Geometry check sheet. Reference: the model listing, model coordinates, mm. A direction names the side the tool comes from. Give positions to 0.01 mm unless a question says otherwise; leave off trailing zeros. Write each loop counter-clockwise with the first axis right and the second up, starting at its lowest first coordinate (ties: lowest second). Pieces come first, ordered by that corner, then holes. Notation, with made-up numbers: M 42.25,-12 L 81.25,-12 A30 cw 81.25,15 Z; hole C 3.5,69.25 d4. An arc over 180 degrees is marked long. One line per item, written item: value. Start each with the question number.
1. Cross-section at A-A on z = 7. Record the cut outline in (x, y).
2. Cross-section at B-B on z = -1.5. Record the cut outline in (x, y).
3. Gauge pin test, flat ends, axial feed: pin 1 (3 mm diameter, centred on y = 48, z = 32, fed in from +X); pin 2 (0.5 mm diameter, centred on x = -1.5, y = 49, fed in from -Z); pin 3 (1.5 mm diameter, centred on y = 50, z = 25, fed in from -X). Record the tip position at first contact, or that the pin passes through.
4. Scan lines: line 1 (Z direction, x = -1.45, y = 48); line 2 (X direction, y = 46.5, z = -1.5); line 3 (Z direction, x = -3.3, y = 48.25). Record each from-to range of solid material in increasing order.
5. Tool access check on faces 1 (the face through (-3.62, 48, -3)), 2 (the face through (-1.968, 48, -3)), 3 (the face through (-3, 50.8, 16)). Record the directions out of +Z, -Z, +X, -X, +Y, -Y that give a thin tool (end or side, any length) a straight path to the whole face; none if there is none.
Autodesk Inventor part; units mm, degrees
ref_plane "Work Plane1" through (0, 50.8, 0) normal (0, 1, 0) x (-1, 0, 0)
ref_plane "YZ Plane" through (0, 0, 0) normal (1, 0, 0) x (0, 1, 0)
ref_plane "XY Plane" through (0, 0, 0) normal (0, 0, 1) x (1, 0, 0)
sketch "Sketch6" plane through (0, 0, 0) normal (0, 1, 0) x (-1, 0, 0)
  line L0 (0, 0) -> (5.588, 0)
  line L1 (5.588, 0) -> (5.588, -6.35)
  line L2 (5.588, -6.35) -> (0, -6.35)
  line L3 (0, -6.35) -> (0, 0)
  arc A0 (0, -6.35) -> (5.588, -6.35) centre (2.794, -6.35) ccw
  dimension "d25" = 5.588
  dimension "d26" = 6.35
ref_plane "Work Plane1" through (0, 50.8, 0) normal (0, 1, 0) x (-1, 0, 0)
sketch "Sketch8" plane through (0, 50.8, 0) normal (0, 1, 0) x (-1, 0, 0)
  line L0 (4.3815, 0) -> (1.2065, 0)
  line L1 (1.2065, 0) -> (1.2065, -3.81)
  line L2 (1.2065, -3.81) -> (4.3815, -3.81)
  line L3 (4.3815, -3.81) -> (4.3815, 0)
  arc A0 (1.2065, -3.81) -> (4.3815, -3.81) centre (2.794, -3.81) ccw
  point P0 (0, 0)
  dimension "d27" = 3.175
  dimension "d28" = 3.81
  dimension "d49" = 1.2065
loft "Loft1" add profiles "Sketch6", "Sketch8"
sketch "Sketch9" plane through (-5.588, 0, 0) normal (0, 0, 1) x (1, 0, 0)
  line L0 (0, 0) -> (5.588, 0)
  line L1 (5.588, 0) -> (4.3815, 50.8)
  line L2 (1.2065, 50.8) -> (4.3815, 50.8)
  line L3 (0, 0) -> (1.2065, 50.8)
  line L4 (4.3815, 50.8) -> (5.588, 0)
  line L5 (4.5323, 44.45) -> (1.0557, 44.45)
  line L6 (0, 0) -> (1.2065, 50.8)
  dimension "d34" = 6.35
extrude "Extrusion5" add sketch "Sketch9" along normal blind 38.608 contours L3 L2 L1 L5
sketch "Sketch12" plane through (-2.794, 0, -6.35) normal (0, -1, 0) x (1, 0, 0)
  circle A0 centre (0, 1.9685) radius 1.27
  arc A1 (-2.794, 0) -> (2.794, 0) centre (0, 0) ccw
  line L0 (0, -2.794) -> (0, 1.9685)
  point P0 (2.794, 6.35)
  dimension "d44" = 2.54
  dimension "d46" = 4.7625
extrude "Extrusion8" cut sketch "Sketch12" against normal blind 10.16
sketch "Sketch13" plane through (-5.588, 0, 0) normal (0, 0, 1) x (1, 0, 0)
  line L0 (4.3815, 50.8) -> (1.2065, 50.8)
  line L1 (1.2065, 50.8) -> (4.3815, 50.8)
  line L2 (1.0557, 44.45) -> (4.5323, 44.45)
  line L3 (3.6195, 50.8) -> (1.9685, 50.8)
  line L4 (1.9685, 50.8) -> (1.9685, 44.45)
  line L5 (1.9685, 44.45) -> (3.6195, 44.45)
  line L6 (3.6195, 44.45) -> (3.6195, 50.8)
  line L7 (3.6195, 50.8) -> (4.3815, 50.8) construction
  line L8 (0, 0) -> (1.2065, 50.8) construction
  line L9 (1.9685, 50.8) -> (1.2065, 50.8) construction
  line L10 (10.7022, 53.5114) -> (-2.6174, 53.5114)
  line L11 (-2.6174, 53.5114) -> (-2.6174, -3.5015)
  line L12 (-2.6174, -3.5015) -> (10.7022, -3.5015)
  line L13 (10.7022, -3.5015) -> (10.7022, 53.5114)
  line L14 (1.9685, 50.8) -> (1.2065, 50.8)
  line L15 (1.2065, 50.8) -> (1.0557, 44.45)
  line L16 (1.9685, 44.45) -> (1.0557, 44.45)
  line L17 (4.3815, 50.8) -> (5.588, 0)
  line L18 (3.6195, 44.45) -> (4.5323, 44.45)
  line L19 (4.5323, 44.45) -> (4.3815, 50.8)
  line L20 (4.3815, 50.8) -> (3.6195, 50.8)
  dimension "d50" = 1.651
extrude "Extrusion11" cut sketch "Sketch13" against normal through all contours L17 L2 L6 L0 | L4 L2 L15 L0
sketch "Sketch15" plane through (-5.588, 0, 0) normal (0, 0, 1) x (1, 0, 0)
  line L0 (8.5653, 44.45) -> (-2.8373, 44.45)
  line L1 (-2.8373, 44.45) -> (-2.8373, 0)
  line L2 (-2.8373, 0) -> (8.5653, 0)
  line L3 (8.5653, 0) -> (8.5653, 44.45)
  point P0 (5.588, 0)
extrude "Extrusion12" cut sketch "Sketch15" against normal through all
properties part number "RudderStabilizingFins_Print2"
Report:
1. outline: M -4.53,44.45 L -1.06,44.45 L -1.21,50.8 L -4.38,50.8 Z
2. outline: M -3.62,44.45 L -1.97,44.45 L -1.97,50.8 L -3.62,50.8 Z
3. pin 1: stops at x = -1.1
3. pin 2: stops at z = 0
3. pin 3: stops at x = -4.42
4. line 1: z = 0 to 38.61
4. line 2: x = -3.62 to -1.97
4. line 3: z = -5.51 to 38.61
5. face 1: -Z, -X, +Y, -Y
5. face 2: -Z, +X, +Y, -Y
5. face 3: +Z, -Z, +X, -X, +Y
